Could you check a few things on this model? Use its own coordinates, in mm. A direction names the side the tool comes from. Coordinates: 2 decimals unless noted, no trailing zeros. Write each loop counter-clockwise with the first axis right and the second up, starting at its lowest first coordinate (ties: lowest second). Pieces come first, ordered by that corner, then holes. Notation, with made-up numbers: (-21.5, 47.25) - (27.5, 47.25) arc R19 cw to (27.5, 82.25) - close; hole circle Ø8 at (88, 89.25). An arc over 180 degrees is marked (long way). Answer as a JSON object with one key per item and string values. Group by question number.
1) Please list where these lines run through material, in increasing order: line 1 along Z through (x, y) = (0, -0.6); line 2 along Y through (x, z) = (-4.75, -6); line 3 along Z through (x, y) = (0, 11.5).
2) If we section it at B-B (y = 5.75): Write out the boundary of the cut face in (x, z).
3) If we section it at A-A (z = -4.5): Write out the boundary of the cut face in (x, y).
4) Will these pins go through, and if not, where does the flat tip stop? pin 1 Ø1.2 at (x, z) = (0, 72.8) entering from +Y; pin 2 Ø1.5 at (x, y) = (-0.5, -2.5) entering from -Z; pin 3 Ø1.6 at (x, z) = (-5, -15) entering from +Y; pin 4 Ø2.5 at (x, z) = (0, -6.7) entering from -Y.
5) On a 3-axis mill with a long thin cutter (end or side, diameter ignored), from which of +Z, -Z, +X, -X, +Y, -Y can I reach the whole of each face in a straight line? I mean faces 5 (the flat face through (-4.4, -4, 13.8)), 6 (the flat face through (0, -1, 11)). Say none if no direction works.
6) We'd pull the mould along Y, two halves only. Please class faces 1 (the flat face through (0, 11, 75)), 2 (the flat face through (6.5, -2, 13)), 3 (the flat face through (0, 12, 74)), 4 (the flat face through (0, 5, 79.802)): released by +Y, released by -Y, zero draft, split by the parting line, or undercut.
```python
from build123d import *

# Parameters (mm, degrees)
F0_W      = 13
F0_H      = 138
F1_DEPTH  = 4
F2_W      = 8
F2_H      = 1
F3_DEPTH  = 136
F4_R      = 1
F5_DEPTH  = 4.001
F6_R      = 1
F7_DEPTH  = 4.001
F8_W      = 13
F8_H      = 2
F9_DEPTH  = 12
F10_W     = 13
F10_H     = 1
F11_DEPTH = 13
F12_R     = 1
F13_DEPTH = 16.001


with BuildPart() as f1:
    # F0 (on Front) → F1 (new body)
    with BuildSketch(Plane.XZ):
        with Locations((0, 12.801612)):
            Rectangle(F0_W, F0_H)
    extrude(amount=F1_DEPTH)

    # F2 (on face) → F3 (cut)
    with BuildSketch(Plane(origin=(0, 0, -56.198388), x_dir=(1, 0, 0), z_dir=(0, 0, -1))):
        with Locations((0, 3.5)):
            Rectangle(F2_W, F2_H)
        Polygon((-5.5, 1), (-4, 1), (4, 1), (5.5, 1), (5.5, 3), (4, 3), (-4, 3), (-5.5, 3), align=None)
    extrude(amount=-F3_DEPTH, mode=Mode.SUBTRACT)

    # F4 (on face) → F5 (cut, through all)
    with BuildSketch(Plane.XZ.offset(4)):
        with Locations((0, -46.198388)):
            Circle(F4_R)
    extrude(amount=-F5_DEPTH, mode=Mode.SUBTRACT)

    # F6 (on face) → F7 (cut, through all)
    with BuildSketch(Plane.XZ.offset(4)):
        with Locations((0, -6.698388)):
            Circle(F6_R)
    extrude(amount=-F7_DEPTH, mode=Mode.SUBTRACT)

    # F8 (on face) → F9 (join)
    with BuildSketch(Plane(origin=(0, 0, 0), x_dir=(-1, 0, 0), z_dir=(0, 1, 0))):
        with Locations((0, 80.801612)):
            Rectangle(F8_W, F8_H)
    extrude(amount=F9_DEPTH)

    # F10 (on face) → F11 (join)
    with BuildSketch(Plane(origin=(0, 0, 79.801612), x_dir=(1, 0, 0), z_dir=(0, 0, -1))):
        with Locations((0, -11.5)):
            Rectangle(F10_W, F10_H)
    extrude(amount=F11_DEPTH)

    # F12 (on face) → F13 (cut, through all)
    with BuildSketch(Plane(origin=(0, 12, 0), x_dir=(-1, 0, 0), z_dir=(0, 1, 0))):
        with Locations((0, 72.801612)):
            Circle(F12_R)
    extrude(amount=-F13_DEPTH, mode=Mode.SUBTRACT)


solid = f1.part
```
Here are the results:
{
 "1": {"line 1": "z = -56.2 to -47.2, -45.2 to -7.7, -5.7 to 71.8, 73.8 to 81.8", "line 2": "y = -4 to -3, -1 to 0", "line 3": "z = 66.8 to 71.8, 73.8 to 81.8"},
 "2": {"outline": "(-6.5, 79.8) - (6.5, 79.8) - (6.5, 81.8) - (-6.5, 81.8) - close"},
 "3": {"outline": "(-6.5, -4) - (-4, -4) - (-4, -3) - (-5.5, -3) - (-5.5, -1) - (5.5, -1) - (5.5, -3) - (4, -3) - (4, -4) - (6.5, -4) - (6.5, 0) - (-6.5, 0) - close"},
 "4": {"pin 1": "passes through", "pin 2": "stops at z = 79.8", "pin 3": "stops at y = 0", "pin 4": "stops at y = -1"},
 "5": {"face 5": "+Z, -Z, +X, -X, -Y", "face 6": "-Z"},
 "6": {"face 1": "undercut", "face 2": "zero draft", "face 3": "released by +Y", "face 4": "undercut"}
}
